from build123d import *

# Parameters (mm, degrees)
BOSS_EXTRUDE1_DEPTH = 150
SKETCH2_W           = 143
SKETCH2_H           = 131
CUT_EXTRUDE1_DEPTH  = 95
SKETCH3_R           = 2.5
BOSS_EXTRUDE2_DEPTH = 1.5
CUT_EXTRUDE2_REACH  = 227.015
SKETCH4_R           = 2.25
SKETCH4_R_2         = 4
SKETCH5_R           = 9
SKETCH5_R_2         = 2.25
SKETCH5_R_3         = 13
SKETCH5_R_4         = 4
BOSS_EXTRUDE3_DEPTH = 4


with BuildPart() as part:
    # Sketch1 → Boss-Extrude1 (new body)
    with BuildSketch(Plane(origin=(0, 0, 0), x_dir=(0, 0, -1), z_dir=(1, 0, 0))):
        with BuildLine():
            Line((0, 0), (-130, 0))
            Line((-130, 0), (-130, 50))
            ThreePointArc((-130, 50), (-115.355339059, 85.355339059), (-80, 100))
            Line((-80, 100), (0, 100))
            Line((0, 100), (0, 0))
        make_face()
    extrude(amount=BOSS_EXTRUDE1_DEPTH)

    # Sketch2 → Cut-Extrude1 (cut)
    with BuildSketch(Plane(origin=(0, 100, 0), x_dir=(1, 0, 0), z_dir=(0, 1, 0))):
        with Locations((75.5, -69.5)):
            Rectangle(SKETCH2_W, SKETCH2_H)
    extrude(amount=-CUT_EXTRUDE1_DEPTH, mode=Mode.SUBTRACT)

    # Sketch3 → Boss-Extrude2 (add, symmetric)
    with BuildSketch(Plane(origin=(111.25, 0, 0), x_dir=(0, 0, -1), z_dir=(1, 0, 0))):
        with BuildLine():
            Line((0, 100), (0, 86.483689179))
            Line((0, 86.483689179), (10.709846007, 98.483689179))
            ThreePointArc((10.709846007, 98.483689179), (10.348889249, 104.837405432), (3.995172996, 104.476448674))
            Line((3.995172996, 104.476448674), (0, 100))
        make_face()
        with Locations((7.352509502, 101.480068927)):
            Circle(SKETCH3_R, mode=Mode.SUBTRACT)
    boss_extrude2 = extrude(amount=BOSS_EXTRUDE2_DEPTH, both=True)

    # Mirror1: Boss-Extrude2 across plane
    add(boss_extrude2.mirror(Plane(origin=(75.5, 0, 0), x_dir=(0, 0, 1), z_dir=(1, 0, 0))))

    # Sketch4 → Cut-Extrude2 (cut, up to next)
    with BuildSketch(Plane(origin=(150, 0, 0), x_dir=(0, 0, -1), z_dir=(1, 0, 0)), mode=Mode.PRIVATE) as cut_extrude2_sk1:
        with Locations((-61.531516432, 29)):
            Circle(SKETCH4_R)
    cut_extrude2_tool1 = extrude(cut_extrude2_sk1.sketch, amount=-CUT_EXTRUDE2_REACH, mode=Mode.PRIVATE) & part.part
    # Sketch4 → Cut-Extrude2 (cut, up to next)
    with BuildSketch(Plane(origin=(150, 0, 0), x_dir=(0, 0, -1), z_dir=(1, 0, 0)), mode=Mode.PRIVATE) as cut_extrude2_sk2:
        with Locations((-7.503745795, 88)):
            Circle(SKETCH4_R_2)
    cut_extrude2_tool2 = extrude(cut_extrude2_sk2.sketch, amount=-CUT_EXTRUDE2_REACH, mode=Mode.PRIVATE) & part.part
    cut_extrude2_1 = cut_extrude2_tool1.solids().sort_by_distance((150, 29, 61.531516))[0]
    add(cut_extrude2_1, mode=Mode.SUBTRACT)
    cut_extrude2_2 = cut_extrude2_tool2.solids().sort_by_distance((150, 88, 7.503746))[0]
    add(cut_extrude2_2, mode=Mode.SUBTRACT)
    cut_extrude2 = cut_extrude2_1 + cut_extrude2_2  # Cut-Extrude2 as one shape, for the pattern or mirror that repeats it

    # Mirror2: Cut-Extrude2 across plane
    add(cut_extrude2.mirror(Plane(origin=(75.5, 0, 0), x_dir=(0, 0, 1), z_dir=(1, 0, 0))), mode=Mode.SUBTRACT)

    # Sketch5 → Boss-Extrude3 (add)
    # profile 1 of 2: a face of its own
    with BuildSketch(Plane(origin=(150, 0, 0), x_dir=(0, 0, -1), z_dir=(1, 0, 0))):
        with Locations(Location((-7.5, 88, 0), (0, 0, 326.442690238))):
            Circle(SKETCH5_R)
        with Locations((-7.5, 88)):
            Circle(SKETCH5_R_2, mode=Mode.SUBTRACT)
    # profile 2 of 2: a face of its own
    with BuildSketch(Plane(origin=(150, 0, 0), x_dir=(0, 0, -1), z_dir=(1, 0, 0))):
        with Locations((-61.53, 29)):
            Circle(SKETCH5_R_3)
        with Locations((-61.53, 29)):
            Circle(SKETCH5_R_4, mode=Mode.SUBTRACT)
    boss_extrude3 = extrude(amount=BOSS_EXTRUDE3_DEPTH)

    # Mirror3: Boss-Extrude3 across plane
    add(boss_extrude3.mirror(Plane(origin=(75.5, 0, 0), x_dir=(0, 0, 1), z_dir=(1, 0, 0))))


solid = part.part
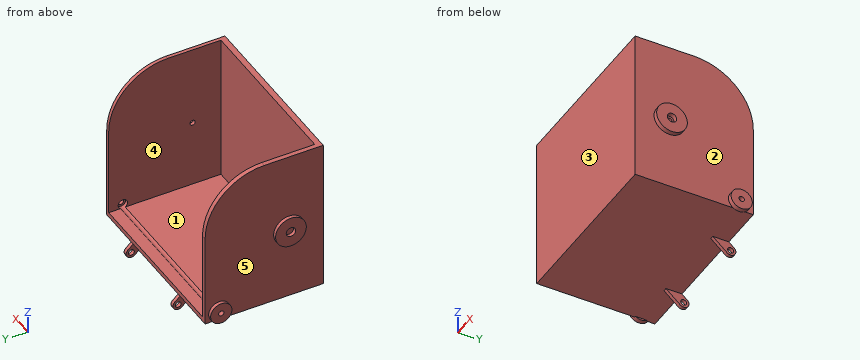
Read the model definition and answer for the solid it produces. Units are mm, in the model's axes. Face numbers are marked on the shaded views. A direction names the side the tool comes from. Coordinates: 2 decimals unless noted, no trailing zeros. Loops run counter-clockwise (first coordinate to the right, second up) from the corner with the lowest first, then second, coordinate; pieces in that order, holes last.
Q1. Each of these flat-tipped pins is pushed along its axis until it touches: pin 1 Ø8 at (x, z) = (126, 75.5) entering from +Y; pin 2 Ø8 at (y, z) = (62.5, 16) entering from +X; pin 3 Ø6 at (y, z) = (93, -5) entering from -X. Where does it stop, or does it pass through?
Q2. Which of the six approach directions +Z, -Z, +X, -X, +Y, -Y give full straight-line access (tool end or side, diameter ignored) to the marked faces 4 and 5?
Q3. The part is cut by section C-C on x = 57. Write down the section's boundary in (y, z), and give its area (3 significant figures).
Q4. Consider probe 1 along Y at (x, z) = (-1.6, 61.53); probe 2 along X at (y, z) = (96, -4.5); probe 3 along X at (y, z) = (21, 114.5). Determine where each line is inside the solid, lowest interval first.
Q5. The part is cut by section B-B on y = 11. Write down the section's boundary in (x, z), and give its area (3 significant figures).
Q6. The part is cut by section A-A on z = 7.5. Give the number of separate pieces and of enclosed holes in the cut face, and give its area (3 significant figures).
Q7. The mould has two halves that part along X. Classify the marked faces 1, 2 and 3: +X half, -X half, draft (parallel to the pull), parting line (faces both ways), or undercut.
Results below:
1. pin 1: stops at y = 5
1. pin 2: stops at x = 150
1. pin 3: stops at x = 38.25
2. face 4: +Z, +Y
2. face 5: -X
3. outline: (0, 0) - (100, 0) - (100, 4) - (89.93, 4) arc R4 cw to (86.07, 4) - (5, 4) - (5, 130) - (0, 130) - close
3. area: 1,030 mm2
4. probe 1: y = 16 to 25, 33 to 42
4. probe 2: x = 38.25 to 41.25, 109.75 to 112.75
4. probe 3: x = 0 to 4, 147 to 150
5. outline: (0, 0) - (150, 0) - (150, 130) - (147, 130) - (147, 4) - (4, 4) - (4, 130) - (0, 130) - close
5. area: 1,480 mm2
6. separate pieces: 3
6. enclosed holes: 0
6. area: 1,460 mm2
7. face 1: undercut
7. face 2: +X half
7. face 3: draft
